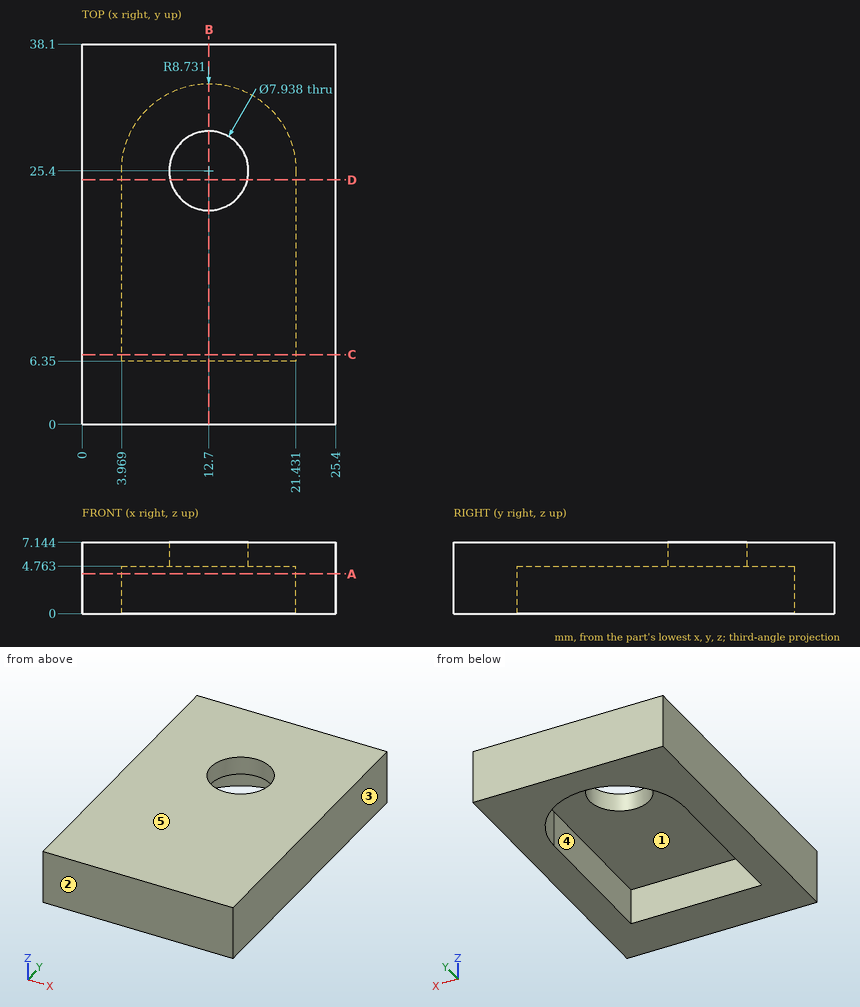
Here's the drawing with two shaded views (mm, measured from the low corner). I have some questions. A direction names the side the tool comes from. Coordinates: 2 decimals unless noted, no trailing zeros. Loops run counter-clockwise (first coordinate to the right, second up) from the corner with the lowest first, then second, coordinate; pieces in that order, holes last. Notation, with made-up numbers: (-38.5, 45) -> (13.5, 45) arc R20 cw to (13.5, 55) -> close; hole circle Ø10 at (-34.75, 14). An arc over 180 degrees is marked (long way). Use one line per item in the form item = value. Start each with the question number.
(1) If we section it at D-D (y = 24.5): Please give me the cut outline in (x, z) (1 decimal).
(2) Will these pins go through, and if not, where does the flat tip stop? pin 1 (1 mm diameter, centred on x = 8.5, y = 29, fed in from -Z); pin 2 (2.5 mm diameter, centred on y = 13.5, z = 3.5, fed in from -X).
(3) If we section it at A-A (z = 4): Please give me the cut outline in (x, y).
(4) We'd pull the mould along X, two halves only. Please class the marked faces 3, 4 and 5: pulls with the +X half, pulls with the -X half, needs draft (parallel to the pull), parting line crosses it, or undercut.
(5) Please list where these lines run through material, in increasing order: line 1 along Y through (x, z) = (12.75, 4); line 2 along X through (y, z) = (21.5, 2); line 3 along Y through (x, z) = (12.7, 5.3).
(6) On a 3-axis mill with a long thin cutter (end or side, diameter ignored), from which of +Z, -Z, +X, -X, +Y, -Y can I reach the whole of each face in a straight line? I mean the marked faces 1 and 2. Say none if no direction works.
(7) If we section it at C-C (y = 7): Please give me the cut outline in (x, z).
(8) If we section it at B-B (x = 12.7): Please give me the cut outline in (y, z), then the cut area to 3 significant figures.
Verdict:
q1.outline = (0, 0) -> (4, 0) -> (4, 4.8) -> (8.8, 4.8) -> (8.8, 7.1) -> (0, 7.1) -> close; (16.6, 4.8) -> (21.4, 4.8) -> (21.4, 0) -> (25.4, 0) -> (25.4, 7.1) -> (16.6, 7.1) -> close
q2.pin_1 = 4.76
q2.pin_2 = 0
q3.outline = (0, 0) -> (25.4, 0) -> (25.4, 38.1) -> (0, 38.1) -> close; hole (3.97, 6.35) -> (21.43, 6.35) -> (21.43, 25.4) arc R8.73 ccw to (3.97, 25.4) -> close
q4.face_3 = pulls with the +X half
q4.face_4 = undercut
q4.face_5 = needs draft
q5.line_1 = 0 to 6.35, 34.13 to 38.1
q5.line_2 = 0 to 3.97, 21.43 to 25.4
q5.line_3 = 0 to 21.43, 29.37 to 38.1
q6.face_1 = -Z
q6.face_2 = +Z, -Z, +X, -X, -Y
q7.outline = (0, 0) -> (3.97, 0) -> (3.97, 4.76) -> (21.43, 4.76) -> (21.43, 0) -> (25.4, 0) -> (25.4, 7.14) -> (0, 7.14) -> close
q8.outline = (0, 0) -> (6.35, 0) -> (6.35, 4.76) -> (21.43, 4.76) -> (21.43, 7.14) -> (0, 7.14) -> close; (29.37, 4.76) -> (34.13, 4.76) -> (34.13, 0) -> (38.1, 0) -> (38.1, 7.14) -> (29.37, 7.14) -> close
q8.area = 121 mm²
